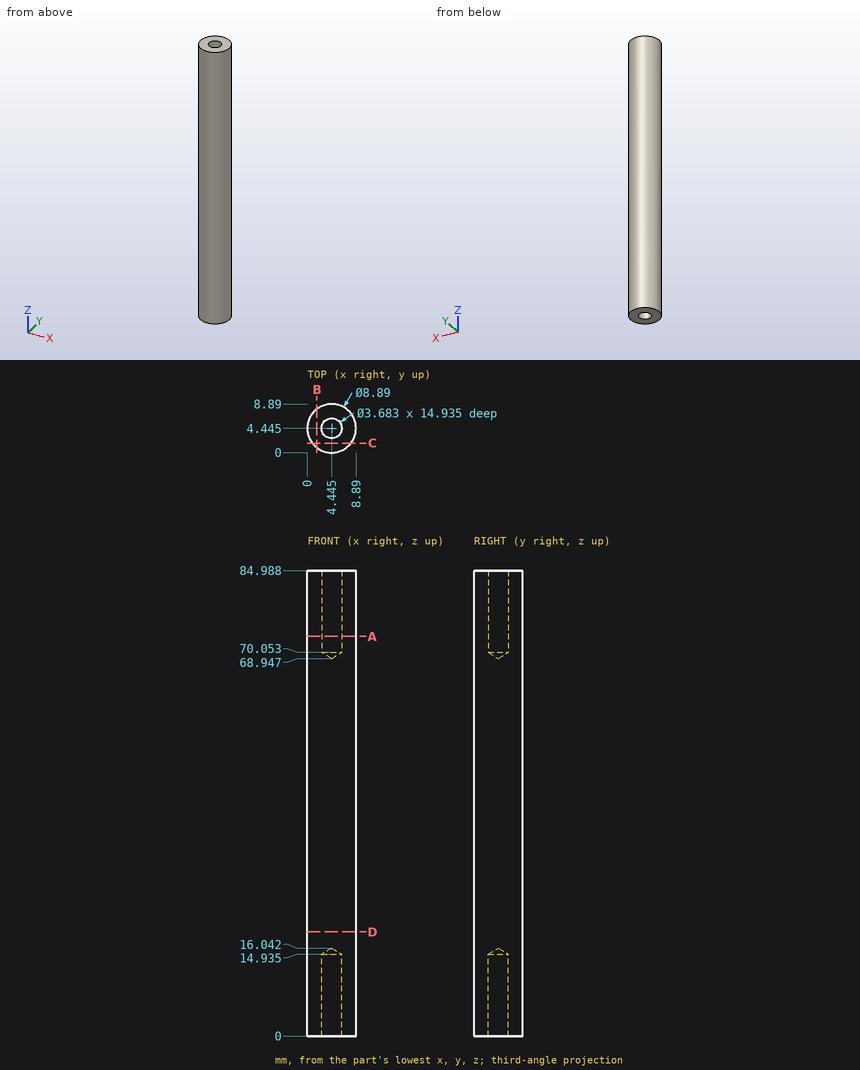
Could you check a few things on this drawing? It's one solid part, dimensions in mm from its lowest x, y, z. Round coordinates to 2 decimals unless told otherwise and drop trailing zeros. Write each loop counter-clockwise with the first axis right and the second up, starting at its lowest first coordinate (ties: lowest second). Pieces come first, ordered by that corner, then holes. Notation, with made-up numbers: M -5.5,-39.75 L 24.5,-39.75 A20 cw 24.5,-31.75 Z; hole C 15.5,26 d5. An arc over 180 degrees is marked long. Answer as CSV lines item,"result". Start each with the question number.
1. Suppose I cut it at D-D on z = 19. Write out the boundary of the cut face in (x, y) (1 decimal).
2. Suppose I cut it at A-A on z = 73. Write out the boundary of the cut face in (x, y) (1 decimal), then the cut area to 3 significant figures.
3. I need wall thicknesses on probe 1 along Y at (x, z) = (4.25, 72.5) (1 decimal); probe 2 along Y at (x, z) = (5.5, 6.5) (1 decimal); probe 3 along X at (y, z) = (6, 9). Which ranges of each line are inside material? Lowest first, please.
4. I'm going to push flat-ended pins straight in: pin 1 Ø4 at (x, y) = (6, 1) entering from -Z; pin 2 Ø4 at (x, z) = (8, 38.5) entering from +Y; pin 3 Ø1 at (y, z) = (2, 27) entering from +X; pin 4 Ø2 at (x, z) = (3, 18.5) entering from -Y. Where does each tip first touch, or does it pass through?
5. Suppose I cut it at B-B on x = 1.75. Write out the boundary of the cut face in (y, z).
Check result:
1,outline,"C 4.4,4.4 d8.9"
2,outline,"C 4.4,4.4 d8.9; hole C 4.4,4.4 d3.7"
2,area,"51.4 mm2"
3,probe 1,"y = 0 to 2.6, 6.3 to 8.9"
3,probe 2,"y = 0.1 to 2.9, 6 to 8.8"
3,probe 3,"x = 0.28 to 3.46, 5.43 to 8.61"
4,pin 1,"stops at z = 0"
4,pin 2,"stops at y = 8.61"
4,pin 3,"stops at x = 8.44"
4,pin 4,"stops at y = 0.02"
5,outline,"M 0.91,0 L 7.98,0 L 7.98,84.99 L 0.91,84.99 Z"
